from build123d import *

# Parameters (mm, degrees)
BOSS_EXTRUDE1_DEPTH = 15
SKETCH2_R           = 10.6
CUT_EXTRUDE1_DEPTH  = 12
SKETCH3_R           = 6.5
CUT_EXTRUDE2_DEPTH  = 10


with BuildPart() as part:
    # Sketch1 → Boss-Extrude1 (new body)
    with BuildSketch(Plane.XY):
        with BuildLine():
            Line((-150, 160), (150, 160))
            ThreePointArc((150, 160), (157.071067812, 157.071067812), (160, 150))
            Line((160, 150), (160, -150))
            ThreePointArc((160, -150), (157.071067812, -157.071067812), (150, -160))
            Line((150, -160), (-150, -160))
            ThreePointArc((-150, -160), (-157.071067812, -157.071067812), (-160, -150))
            Line((-160, -150), (-160, 150))
            ThreePointArc((-160, 150), (-157.071067812, 157.071067812), (-150, 160))
        make_face()
    extrude(amount=BOSS_EXTRUDE1_DEPTH)

    # Sketch2 → Cut-Extrude1 (cut)
    with BuildSketch(Plane.XY.offset(15)):
        Circle(SKETCH2_R)
    extrude(amount=-CUT_EXTRUDE1_DEPTH, mode=Mode.SUBTRACT)

    # Sketch3 → Cut-Extrude2 (cut)
    with BuildSketch(Plane.XY.offset(3)):
        Circle(SKETCH3_R)
    extrude(amount=-CUT_EXTRUDE2_DEPTH, mode=Mode.SUBTRACT)


solid = part.part
Verification items for the finished model (mm, model axes). A direction names the side the tool comes from. Coordinates: 2 decimals unless noted, no trailing zeros. Write each loop counter-clockwise with the first axis right and the second up, starting at its lowest first coordinate (ties: lowest second). Pieces come first, ordered by that corner, then holes. Notation, with made-up numbers: (6, -31.5) -> (10, -31.5) arc R25 cw to (10, -14.5) -> close; hole circle Ø10 at (18, -4). An arc over 180 degrees is marked (long way). One line per item, written item: value. Start each with the question number.
Q1. Access from +Z, -Z, +X, -X, +Y, -Y to the whole of each face (thin tool, end or side, straight path). Record for faces 4 (the cylindrical face through (156.99, 157.15, 7.4)), 5 (the flat face through (5, 5, 3)).
Q2. Thickness scan on L1, parallel to Y at x = 0, z = 1.55; L2, parallel to Y at x = 0, z = 12. Record the ranges inside material, lowest first. Write a range as from..to.
Q3. Mould release check, pull along X, two halves, no side actions. Record for faces 1 (the flat face through (-160, -2, 7)), 2 (the flat face through (160, 2, 7)), 3 (the cylindrical face through (9.79, -4.06, 9.08)): pulls with the +X half, pulls with the -X half, needs draft (parallel to the pull), parting line crosses it, or undercut.
Q4. Cross-section at A-A on y = 0. Enter the section's corners in (x, z).
Q5. Go/stop test with flat-tipped pins: P1, Ø6.5, axis at x = -3.5, y = 5, coming from the +Z side; P2, Ø10.5, axis at x = 0, y = 0, coming from the -Z side. Record where each tip stops, or that it passes through.
Checked values:
1. face 4: +Z, -Z, +X, +Y
1. face 5: +Z
2. L1: y = -160..-6.5, 6.5..160
2. L2: y = -160..-10.6, 10.6..160
3. face 1: pulls with the -X half
3. face 2: pulls with the +X half
3. face 3: undercut
4. outline: (-160, 0) -> (-6.5, 0) -> (-6.5, 3) -> (-10.6, 3) -> (-10.6, 15) -> (-160, 15) -> close; (6.5, 0) -> (160, 0) -> (160, 15) -> (10.6, 15) -> (10.6, 3) -> (6.5, 3) -> close
5. P1: stops at z = 3
5. P2: passes through
